from build123d import *

# Parameters (mm, degrees)
F0_W     = 147.6248
F0_H     = 62.992
F0_W_2   = 130.3528
F0_H_2   = 55.88
F1_DEPTH = 1.778
F2_W     = 8.128
F2_H     = 55.88
F3_DEPTH = 1.27
F4_W     = 30.776053
F4_H     = 7.62
F5_DEPTH = 1.778
F7_W     = 5.00126
F7_H     = 7.62
F7_W_2   = 5.0038
F8_DEPTH = 6.223
F9_R     = 2.4384
F10_R    = 2.4384


with BuildPart() as f1:
    # F0 (on Front) → F1 (new body)
    with BuildSketch(Plane.XZ):
        Rectangle(F0_W, F0_H)
        Rectangle(F0_W_2, F0_H_2, mode=Mode.SUBTRACT)
    extrude(amount=F1_DEPTH)

    # F2 (on face) → F3 (join)
    with BuildSketch(Plane.XZ.offset(1.778)):
        with Locations((-55.39232, 0)):
            Rectangle(F2_W, F2_H)
        with Locations((-41.54424, 0)):
            Rectangle(F2_W, F2_H)
        with Locations((-27.69616, 0)):
            Rectangle(F2_W, F2_H)
        with Locations((-13.84808, 0)):
            Rectangle(F2_W, F2_H)
        Rectangle(F2_W, F2_H)
        with Locations((13.84808, 0)):
            Rectangle(F2_W, F2_H)
        with Locations((27.69616, 0)):
            Rectangle(F2_W, F2_H)
        with Locations((41.54424, 0)):
            Rectangle(F2_W, F2_H)
        with Locations((55.39232, 0)):
            Rectangle(F2_W, F2_H)
    extrude(amount=-F3_DEPTH)

    # F4 (on face) → F5 (join)
    with BuildSketch(Plane.XZ.offset(1.778)):
        with Locations((-80.564426, 23.279527)):
            Rectangle(F4_W, F4_H)
    extrude(amount=-F5_DEPTH)

    # F7 (on face) → F8 (join)
    with BuildSketch(Plane.XZ.offset(1.778)):
        with Locations((-89.788674, 23.279527)):
            Rectangle(F7_W, F7_H)
        with Locations((-78.791744, 23.279527)):
            Rectangle(F7_W_2, F7_H)
    extrude(amount=F8_DEPTH)

    # F9
    f9_edges = [f1.edges().sort_by_distance(p)[0] for p in [
        (-87.288044, -8.001, 23.279527),
        (-89.788674, -8.001, 27.089527),
        (-92.289304, -8.001, 23.279527),
        (-89.788674, -8.001, 19.469527),
    ]]
    fillet(f9_edges, radius=F9_R)

    # F10
    f10_edges = [f1.edges().sort_by_distance(p)[0] for p in [
        (-78.791744, -8.001, 27.089527),
        (-81.293644, -8.001, 23.279527),
        (-78.791744, -8.001, 19.469527),
        (-76.289844, -8.001, 23.279527),
    ]]
    fillet(f10_edges, radius=F10_R)


solid = f1.part
Build history of the part. All positions in model axes, mm. A direction names the side the tool comes from. Give positions to 0.01 mm unless a question says otherwise; leave off trailing zeros. Loops run counter-clockwise (first coordinate to the right, second up) from the corner with the lowest first, then second, coordinate; pieces in that order, holes last. Notation, with made-up numbers: (83.25, -14) - (121.25, -14) arc R9 cw to (121.25, -6) - close; hole circle Ø9 at (78, 30.5). An arc over 180 degrees is marked (long way). Write item = value, one per line. Start each with the question number.
1) Drop flat-ended pins along their axis: pin 1 Ø9 at (x, z) = (26.5, -11) entering from +Y; pin 2 Ø5 at (x, z) = (-85.5, 21.5) entering from -Y; pin 3 Ø1 at (y, z) = (-1.5, -6.5) entering from -X. Give the stop position or say it passes through.
2) Band-saw the part on A-A on x = -21. Give the cut face in (y, z), plus the area to 3 significant figures.
3) Tool access for faces 5 (the flat face through (-85, -1.6, 27.09)), 6 (the flat face through (-55, -0.508, 0)), 7 (the flat face through (-94, -1.778, 23)), 8 (the flat face through (-81.294, -4, 23)): list every direction of +Z, -Z, +X, -X, +Y, -Y with a clear straight run to the whole face (end or side of a thin tool).
4) Band-saw the part on C-C on z = -14. Count the separate pieces of the cut face and the enclosed holes in it, plus the area to 3 significant figures.
5) Probe probe 1 along X at (y, z) = (-4.5, 22); probe 2 along Z at (x, y) = (32.5, -0.25); probe 3 along X at (y, z) = (-0.25, -1). List the from-to ranges inside material, lowest first. Write a range as from..to.
6) Pull direction X, two halves, no side cores. Call faces 1 (the flat face through (-76.29, -4, 23)), 2 (the flat face through (-85, -1.6, 19.47)), 3 (the flat face through (-28, -0.508, 0)), 4 (the flat face through (-92.289, -4, 23)): +X half, -X half, draft (parallel to the pull), parting line (faces both ways), or undercut.
7) Band-saw the part on B-B on y = -3. Give the cut face in (x, z), plus the area to 3 significant figures.
Final values:
q1.pin_1 = -0.51
q1.pin_2 = -7.28
q1.pin_3 = -73.81
q2.outline = (-1.78, -31.5) - (0, -31.5) - (0, -27.94) - (-1.78, -27.94) - close; (-1.78, 27.94) - (0, 27.94) - (0, 31.5) - (-1.78, 31.5) - close
q2.area = 12.6 mm²
q3.face_5 = +Z, -X, +Y, -Y
q3.face_6 = +Y
q3.face_7 = +Z, -Z, -X, -Y
q3.face_8 = +Z, -Z, -Y
q4.separate_pieces = 11
q4.enclosed_holes = 0
q4.area = 124 mm²
q5.probe_1 = -92.29..-87.29, -81.29..-76.29
q5.probe_2 = -31.5..-27.94, 27.94..31.5
q5.probe_3 = -73.81..-65.18, 65.18..73.81
q6.face_1 = +X half
q6.face_2 = draft
q6.face_3 = undercut
q6.face_4 = -X half
q7.outline = (-92.29, 19.47) - (-87.29, 19.47) - (-87.29, 27.09) - (-92.29, 27.09) - close; (-81.29, 19.47) - (-76.29, 19.47) - (-76.29, 27.09) - (-81.29, 27.09) - close
q7.area = 76.2 mm²
